Autodesk Inventor part; units mm, degrees
ref_plane "dp1_XY" through (9.525, 5.5309, 0) normal (0, 0, 1) x (1, 0, 0)
ref_plane "dp1_YZ" through (9.525, 5.5309, 0) normal (1, 0, 0) x (0, 1, 0)
ref_plane "dp1_ZX" through (9.525, 5.5309, 0) normal (0, 1, 0) x (0, 0, 1)
sketch "Sketch_2" plane through (0, 0, 0) normal (0, 0, 1) x (1, 0, 0)
  line L0 (9.525, 0) -> (0, 0)
  line L1 (0, 0) -> (0, 4.8006)
  line L2 (0, 4.8006) -> (0.7556, 5.5563)
  line L3 (0.7556, 5.5563) -> (4.6603, 5.5563)
  line L4 (4.6603, 5.5563) -> (5.4181, 4.8042)
  arc A0 (5.4181, 4.8042) -> (5.9817, 4.572) centre (5.9817, 5.3721) ccw
  line L5 (5.9817, 4.572) -> (7.1501, 4.572)
  arc A1 (7.1501, 4.572) -> (7.9502, 5.3721) centre (7.1501, 5.3721) ccw
  line L6 (7.9502, 5.3721) -> (7.9502, 5.5309)
  line L7 (7.9502, 5.5309) -> (9.525, 5.5309)
  line L8 (9.525, 5.5309) -> (9.525, 0)
  line L9 (9.525, 0) -> (0, 0)
revolve "Revolution1" add sketch "Sketch_2" angle 360 about axis through (9.525, 0, 0) along (1, 0, 0)
thread "Thread1"
sketch "Sketch_3" plane through (0, 0, 0) normal (0, 0, 1) x (1, 0, 0)
  line L0 (29.3624, 0) -> (9.525, 0)
  line L1 (9.525, 0) -> (9.525, 7.0485)
  line L2 (9.525, 7.0485) -> (10.287, 7.8105)
  line L3 (10.287, 7.8105) -> (25.1206, 7.8105)
  line L4 (25.1206, 7.8105) -> (25.3746, 7.5565)
  line L5 (25.3746, 7.5565) -> (25.3746, 6.6357)
  line L6 (25.3746, 6.6357) -> (26.0096, 6.6357)
  line L7 (26.0096, 6.6357) -> (26.6446, 7.2708)
  line L8 (26.6446, 7.2708) -> (28.8544, 7.2708)
  line L9 (28.8544, 7.2708) -> (29.3624, 6.7627)
  line L10 (29.3624, 6.7627) -> (29.3624, 0)
  line L11 (29.3624, 0) -> (9.525, 0)
revolve "Revolution2" add sketch "Sketch_3" angle 360 about axis through (29.3624, 0, 0) along (1, 0, 0)
sketch "Sketch3" plane through (0, 0, 0) normal (-1, 0, 0) x (0, 0, 1)
  point P0 (0, 0)
hole "Hole1" at (0, 0, 0) direction (1, 0, 0) diameter 4.826 depth 29.3624 countersink diameter 5.842 countersink angle 90
sketch "Sketch_12" plane through (0, 0, 0) normal (0, 1, 0) x (-1, 0, 0)
  line L0 (-19.05, 7.8105) -> (-19.05, -1.016)
  line L1 (-19.05, -1.016) -> (-21.0337, -1.016)
  line L2 (-21.0337, -1.016) -> (-21.0337, 6.3652)
  line L3 (-21.0337, 6.3652) -> (-21.463, 6.7945)
  line L4 (-21.463, 6.7945) -> (-23.0124, 6.7945)
  line L5 (-23.0124, 6.7945) -> (-23.0124, 7.8105)
  line L6 (-23.0124, 7.8105) -> (-19.05, 7.8105)
  line L7 (-19.05, 7.8105) -> (-19.05, -1.016)
revolve "Revolution3" cut sketch "Sketch_12" angle 360 about axis through (19.05, 0, 7.8105) along (0, 0, 1)
thread "Thread2"
sketch "Sketch_47" plane through (0, 0, 0) normal (0, 0, 1) x (1, 0, 0)
  line L0 (26.0096, 0) -> (25.3746, 0)
  line L1 (25.3746, 7.1861) -> (25.3746, 6.3817)
  line L2 (25.3746, 6.3817) -> (26.0096, 6.3817)
  line L3 (26.0096, 6.3817) -> (26.0096, 6.6357)
  line L4 (26.0096, 6.6357) -> (25.6921, 6.6357)
  line L5 (25.6921, 6.6357) -> (25.4916, 6.8362)
  arc A0 (25.4916, 7.0158) -> (25.4916, 6.8362) centre (25.5814, 6.926) ccw
  line L6 (25.4916, 7.0158) -> (26.2022, 7.7263)
  line L7 (26.2022, 7.7263) -> (26.2022, 7.8105)
  line L8 (26.2022, 7.8105) -> (25.999, 7.8105)
  line L9 (25.999, 7.8105) -> (25.3746, 7.1861)
revolve "Revolution4" add sketch "Sketch_47" angle 360 about axis through (26.0096, 0, 0) along (1, 0, 0)
ref_plane "dp1_XY" through (9.525, 5.5309, 0) normal (0, 0, 1) x (1, 0, 0)
ref_plane "dp1_YZ" through (9.525, 5.5309, 0) normal (1, 0, 0) x (0, 1, 0)
ref_plane "dp1_ZX" through (9.525, 5.5309, 0) normal (0, 1, 0) x (0, 0, 1)
ref_plane "dp2_XY" through (9.525, -5.5309, 0) normal (0, 0, 1) x (1, 0, 0)
ref_plane "dp2_YZ" through (9.525, -5.5309, 0) normal (1, 0, 0) x (0, 1, 0)
ref_plane "dp2_ZX" through (9.525, -5.5309, 0) normal (0, 1, 0) x (0, 0, 1)
ref_plane "hh_XY" through (0, 5.5563, 0) normal (0, 0, 1) x (1, 0, 0)
ref_plane "hh_YZ" through (0, 5.5563, 0) normal (1, 0, 0) x (0, 1, 0)
ref_plane "hh_ZX" through (0, 5.5563, 0) normal (0, 1, 0) x (0, 0, 1)
ref_plane "port_XY" through (19.05, 0, 0) normal (0, 0, 1) x (1, 0, 0)
ref_plane "port_YZ" through (19.05, 0, 0) normal (1, 0, 0) x (0, 1, 0)
ref_plane "port_ZX" through (19.05, 0, 0) normal (0, 1, 0) x (0, 0, 1)
ref_plane "rod_guide_XY" through (0, 0, 0) normal (1, 0, 0) x (0, 0, -1)
ref_plane "rod_guide_YZ" through (0, 0, 0) normal (0, 0, -1) x (0, 1, 0)
ref_plane "rod_guide_ZX" through (0, 0, 0) normal (0, 1, 0) x (1, 0, 0)
ref_plane "s1_XY" through (7.9502, 0, 0) normal (0, 0, 1) x (1, 0, 0)
ref_plane "s1_YZ" through (7.9502, 0, 0) normal (1, 0, 0) x (0, 1, 0)
ref_plane "s1_ZX" through (7.9502, 0, 0) normal (0, 1, 0) x (0, 0, 1)
ref_plane "s2_XY" through (9.525, 0, 0) normal (0, 0, 1) x (1, 0, 0)
ref_plane "s2_YZ" through (9.525, 0, 0) normal (1, 0, 0) x (0, 1, 0)
ref_plane "s2_ZX" through (9.525, 0, 0) normal (0, 1, 0) x (0, 0, 1)
ref_plane "t1_XY" through (9.525, 0, 0) normal (1, 0, 0) x (0, 0, -1)
ref_plane "t1_YZ" through (9.525, 0, 0) normal (0, 0, -1) x (0, 1, 0)
ref_plane "t1_ZX" through (9.525, 0, 0) normal (0, 1, 0) x (1, 0, 0)
ref_plane "t111_XY" through (9.525, 0, 0) normal (1, 0, 0) x (0, 0, -1)
ref_plane "t111_YZ" through (9.525, 0, 0) normal (0, 0, -1) x (0, 1, 0)
ref_plane "t111_ZX" through (9.525, 0, 0) normal (0, 1, 0) x (1, 0, 0)
ref_plane "to_foot_bracket_XY" through (9.525, 0, 0) normal (1, 0, 0) x (0, 0, -1)
ref_plane "to_foot_bracket_YZ" through (9.525, 0, 0) normal (0, 0, -1) x (0, 1, 0)
ref_plane "to_foot_bracket_ZX" through (9.525, 0, 0) normal (0, 1, 0) x (1, 0, 0)
ref_plane "to_nut_XY" through (7.9502, 0, 0) normal (1, 0, 0) x (0, 0, -1)
ref_plane "to_nut_YZ" through (7.9502, 0, 0) normal (0, 0, -1) x (0, 1, 0)
ref_plane "to_nut_ZX" through (7.9502, 0, 0) normal (0, 1, 0) x (1, 0, 0)
ref_plane "to_rod_XY" through (0, 0, 0) normal (1, 0, 0) x (0, 0, -1)
ref_plane "to_rod_YZ" through (0, 0, 0) normal (0, 0, -1) x (0, 1, 0)
ref_plane "to_rod_ZX" through (0, 0, 0) normal (0, 1, 0) x (1, 0, 0)
ref_plane "to_screw_XY" through (19.05, 0, 0) normal (0, 1, 0) x (1, 0, 0)
ref_plane "to_screw_YZ" through (19.05, 0, 0) normal (1, 0, 0) x (0, 0, -1)
ref_plane "to_screw_ZX" through (19.05, 0, 0) normal (0, 0, -1) x (0, 1, 0)
ref_plane "to_trunnion_brackets_XY" through (0, 0, 0) normal (0, 1, 0) x (1, 0, 0)
ref_plane "to_trunnion_brackets_YZ" through (0, 0, 0) normal (1, 0, 0) x (0, 0, -1)
ref_plane "to_trunnion_brackets_ZX" through (0, 0, 0) normal (0, 0, -1) x (0, 1, 0)
ref_plane "to_trunnion_brackets1_XY" through (0, 0, 0) normal (0, 1, 0) x (1, 0, 0)
ref_plane "to_trunnion_brackets1_YZ" through (0, 0, 0) normal (1, 0, 0) x (0, 0, -1)
ref_plane "to_trunnion_brackets1_ZX" through (0, 0, 0) normal (0, 0, -1) x (0, 1, 0)
ref_plane "to_trunnion_brackets2_XY" through (0, 0, 0) normal (0, 1, 0) x (1, 0, 0)
ref_plane "to_trunnion_brackets2_YZ" through (0, 0, 0) normal (1, 0, 0) x (0, 0, -1)
ref_plane "to_trunnion_brackets2_ZX" through (0, 0, 0) normal (0, 0, -1) x (0, 1, 0)
ref_plane "to_tube_XY" through (26.0096, 0, 0) normal (1, 0, 0) x (0, 0, -1)
ref_plane "to_tube_YZ" through (26.0096, 0, 0) normal (0, 0, -1) x (0, 1, 0)
ref_plane "to_tube_ZX" through (26.0096, 0, 0) normal (0, 1, 0) x (1, 0, 0)
properties part number "02R000-0_rod_guide"
Work out the finished part from the listing and answer in its coordinate system (mm). A direction names the side the tool comes from. Give positions to 0.01 mm unless a question says otherwise; leave off trailing zeros. Write each loop counter-clockwise with the first axis right and the second up, starting at its lowest first coordinate (ties: lowest second). Pieces come first, ordered by that corner, then holes. Notation, with made-up numbers: (15.25, 26.25) - (40.25, 26.25) arc R22 ccw to (40.25, 50.25) - close; hole circle Ø9 at (73, 78.25). An arc over 180 degrees is marked (long way). One line per item, written item: value. Start each with the question number.
1. Find section D-D (x = 24.5). Write down the section's boundary in (y, z).
2. Find section A-A (x = 19.05). Write down the section's boundary in (y, z), then the cut area to 3 significant figures.
3. For a pull along X with two mould halves and no side action, classify faces 3 (the cylindrical face through (23.01, -0.07, 7.2)), 4 (the cylindrical face through (27.765, -5.77, -4.424)), 5 (the flat face through (0, -0.1, -3.1)) as +X half, -X half, draft (parallel to the pull), parting line (faces both ways), or undercut.
4. Find section C-C (y = -1). State how many separate pieces and enclosed holes the cut face has, then the cut area to 3 significant figures.
5. Given pin 1 (1 mm diameter, centred on x = 15.5, z = 4.5, fed in from +Y); pin 2 (2.5 mm diameter, centred on x = 19.5, y = 0, fed in from +Z); pin 3 (4 mm diameter, centred on x = 4, z = 3.5, fed in from -Y); pin 4 (4 mm diameter, centred on y = 0, z = 0, fed in from +X), each flat-ended and moving along its own axis, determine where each tip first touches the part or whether it passes through.
6. Find section B-B (x = 4). Write down the section's boundary in (y, z), then the cut area to 3 significant figures.
7. For faces 1 (the cylindrical face through (17.808, -1.693, -7.625)), 2 (the cylindrical face through (15.09, 0.07, 7.2)), determine the directions among +Z, -Z, +X, -X, +Y, -Y from which every point of the face is accessible in a straight line to the end or side of a thin tool.
8. Consider probe 1 along Z at (x, y) = (9.25, 0); probe 2 along X at (y, z) = (0, 3.7); probe 3 along X at (y, z) = (0, 4.65). Determine where each line is inside the solid, lowest interval first.
Geometry results:
1. outline: circle Ø15.62 at (0, 0); hole circle Ø4.83 at (0, 0)
2. outline: (-3.85, 6.79) arc R7.81 ccw (long way) to (3.85, 6.79) - (2.41, 6.79) - (1.98, 6.37) - (1.98, 1.37) arc R2.41 cw (long way) to (-1.98, 1.37) - (-1.98, 6.37) - (-2.41, 6.79) - close
2. area: 149 mm2
3. face 3: undercut
3. face 4: draft
3. face 5: -X half
4. separate pieces: 3
4. enclosed holes: 0
4. area: 247 mm2
5. pin 1: y = 6.71
5. pin 2: z = -2.06
5. pin 3: y = -5.35
5. pin 4: through
6. outline: circle Ø11.11 at (0, 0); hole circle Ø4.83 at (0, 0)
6. area: 78.7 mm2
7. face 1: +X, -X
7. face 2: +Z
8. probe 1: -5.53 to -2.41, 2.41 to 5.53
8. probe 2: 0 to 17.07, 21.03 to 29.36
8. probe 3: 0 to 5.64, 7.49 to 17.07, 21.03 to 29.36
